The listing builds one solid part. Answer for the finished solid, in the listing's coordinates (mm). A direction names the side the tool comes from. Coordinates: 2 decimals unless noted, no trailing zeros. Loops run counter-clockwise (first coordinate to the right, second up) from the corner with the lowest first, then second, coordinate; pieces in that order, holes last. Notation, with made-up numbers: M -12.75,-18.5 L 18.25,-18.5 A9 ccw 18.25,-13.5 Z; hole C 45.5,-33 d9. An arc over 180 degrees is marked long. Answer as a JSON object with one key per item and string values. Group by question number.
1. Given pin 1 (6 mm diameter, centred on y = 8, z = -30, fed in from +X); pin 2 (19 mm diameter, centred on x = 25.5, y = 24.5, fed in from -Z), each flat-ended and moving along its own axis, determine where each tip first touches the part or whether it passes through.
2. Straight lines are drawn through the part: L1, parallel to Y at x = 4, z = -30; L2, parallel to X at y = 17, z = -19.5; L3, parallel to X at y = 14, z = 4. For each, find the intervals that lie inside material, in ascending order.
3. Determine the mould class of faces 1 (the face through (3.94, 5.56, -30.54)), 2 (the face through (20, 19, 8)), 3 (the face through (52, 19, 4)), 4 (the face through (23.6, 23.5, 0)) for opening direction Z: released by +Z, released by -Z, zero draft, split by the parting line, or undercut.
4. For faces 5 (the face through (8, 19, -21)), 6 (the face through (3.94, 31.69, -31.84)), determine the directions among +Z, -Z, +X, -X, +Y, -Y from which every point of the face is accessible in a straight line to the end or side of a thin tool.
5. A cutting plane is placed at A-A on x = 7. Give the vertices of the cut face in (y, z), and give its area (3 significant figures).
6. A cutting plane is placed at D-D on y = 35. Give the vertices of the cut face in (x, z), and give its area (3 significant figures).
7. A cutting plane is placed at B-B on z = -8. Give the vertices of the cut face in (x, y).
8. A cutting plane is placed at C-C on y = 19. Give the vertices of the cut face in (x, z), and give its area (3 significant figures).
from build123d import *

# Parameters (mm, degrees)
SKETCH1_W        = 52
SKETCH1_H        = 38
SKETCH1_R        = 11.1125
FACEUP_DEPTH     = 8
SKETCH8_W        = 8
SKETCH8_H        = 38
FACEDOWN_DEPTH   = 38
FILLET1_R        = 5
SKETCH9_R        = 2.5
SCREWHOLES_DEPTH = 8


with BuildPart() as part:
    # Sketch1 → FaceUp (new body)
    with BuildSketch(Plane.XY):
        with Locations((26, 19)):
            Rectangle(SKETCH1_W, SKETCH1_H)
        with Locations((34, 19)):
            Circle(SKETCH1_R, mode=Mode.SUBTRACT)
    extrude(amount=FACEUP_DEPTH)

    # Sketch8 → FaceDown (add)
    with BuildSketch(Plane(origin=(0, 0, 0), x_dir=(-1, 0, 0), z_dir=(0, 0, -1))):
        with Locations((-4, 19)):
            Rectangle(SKETCH8_W, SKETCH8_H)
    extrude(amount=FACEDOWN_DEPTH)

    # Fillet1
    fillet1_edges = [part.edges().sort_by_distance(p)[0] for p in [
        (8, 19, 0),
    ]]
    fillet(fillet1_edges, radius=FILLET1_R)

    # Sketch9 → ScrewHoles (cut)
    with BuildSketch(Plane.ZY):
        with Locations((-8, 30)):
            Circle(SKETCH9_R)
        with Locations((-30, 30)):
            Circle(SKETCH9_R)
        with Locations((-8, 8)):
            Circle(SKETCH9_R)
        with Locations((-30, 8)):
            Circle(SKETCH9_R)
    extrude(amount=-SCREWHOLES_DEPTH, mode=Mode.SUBTRACT)


solid = part.part
From the geometry:
{
 "1": {"pin 1": "stops at x = 8", "pin 2": "stops at z = 0"},
 "2": {"L1": "y = 0 to 5.5, 10.5 to 27.5, 32.5 to 38", "L2": "x = 0 to 8", "L3": "x = 0 to 24.08, 43.92 to 52"},
 "3": {"face 1": "undercut", "face 2": "released by +Z", "face 3": "zero draft", "face 4": "released by -Z"},
 "4": {"face 5": "-Z, +X, +Y, -Y", "face 6": "+X, -X"},
 "5": {"outline": "M 0,-38 L 38,-38 L 38,8 L 0,8 Z; hole C 8,-30 d5; hole C 8,-8 d5; hole C 30,-30 d5; hole C 30,-8 d5", "area": "1,670 mm²"},
 "6": {"outline": "M 0,-38 L 8,-38 L 8,-5 A5 cw 13,0 L 52,0 L 52,8 L 0,8 Z", "area": "725 mm²"},
 "7": {"outline": "M 0,0 L 8,0 L 8,5.5 L 0,5.5 Z; M 0,10.5 L 8,10.5 L 8,27.5 L 0,27.5 Z; M 0,32.5 L 8,32.5 L 8,38 L 0,38 Z"},
 "8": {"outline": "M 0,-38 L 8,-38 L 8,-5 A5 cw 13,0 L 22.89,0 L 22.89,8 L 0,8 Z; M 45.11,0 L 52,0 L 52,8 L 45.11,8 Z", "area": "548 mm²"}
}
